The listing builds one solid part. Answer for the finished solid, in the listing's coordinates (mm). Face numbers are marked on the shaded views. A direction names the side the tool comes from. Round coordinates to 2 decimals unless told otherwise and drop trailing zeros. Loops run counter-clockwise (first coordinate to the right, second up) from the corner with the lowest first, then second, coordinate; pieces in that order, holes last. Notation, with made-up numbers: (11.25, 58) -> (49.25, 58) arc R24 ccw to (49.25, 96) -> close; hole circle Ø5 at (-2, 78.5). An arc over 180 degrees is marked (long way). One line per question, with ' | ' between items.
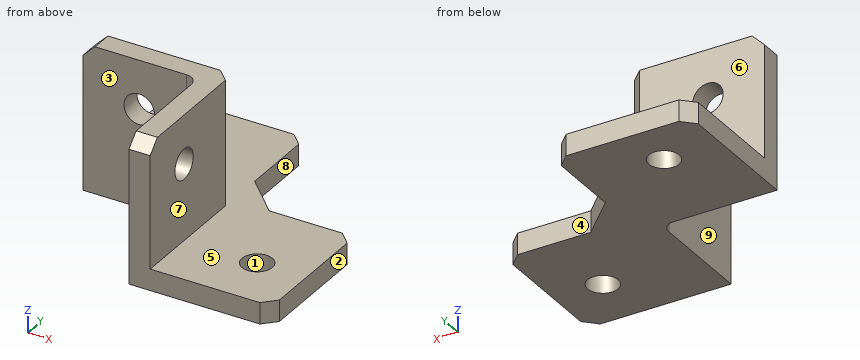
from build123d import *

# Parameters (mm, degrees)
ESQUISSE1_W             = 3.5
ESQUISSE1_H             = 3.5
BOSS_EXTRU_1_DEPTH      = 3.5
ESQUISSE2_W             = 19
ESQUISSE2_H             = 3.5
ESQUISSE2_W_2           = 3.5
ESQUISSE2_H_2           = 19
BOSS_EXTRU_2_DEPTH      = 20.5
ESQUISSE3_R             = 2.5
ENL_V_MAT_EXTRU_2_DEPTH = 3.5
ESQUISSE4_R             = 2.5
ENL_V_MAT_EXTRU_3_DEPTH = 3.5
ESQUISSE5_R             = 2.5
ENL_V_MAT_EXTRU_4_DEPTH = 3.5
ESQUISSE6_R             = 2.5
ENL_V_MAT_EXTRU_5_DEPTH = 3.5
CHANFREIN1_SIZE         = 6
CHANFREIN2_SIZE         = 2
CHANFREIN3_SIZE         = 2
CONG_1_R                = 2


with BuildPart() as part:
    # Esquisse1 → Boss.-Extru.1 (new body)
    with BuildSketch(Plane.XY):
        Polygon((-23.276688067, 13.678057554), (-45.776688067, 13.678057554), (-45.776688067, -9.821942446), (-26.776688067, -9.821942446), (-26.776688067, -6.321942446), (-23.276688067, -6.321942446), align=None)
        with Locations((-25.026688067, -8.071942446)):
            Rectangle(ESQUISSE1_W, ESQUISSE1_H)
        Polygon((-3.276688067, -6.321942446), (-23.276688067, -6.321942446), (-23.276688067, -9.821942446), (-26.776688067, -9.821942446), (-26.776688067, -28.821942446), (-3.276688067, -28.821942446), align=None)
    extrude(amount=BOSS_EXTRU_1_DEPTH)

    # Esquisse2 → Boss.-Extru.2 (add)
    with BuildSketch(Plane.XY.offset(3.5)):
        with Locations((-36.276688067, -8.071942446)):
            Rectangle(ESQUISSE2_W, ESQUISSE2_H)
        with Locations((-25.026688067, -8.071942446)):
            Rectangle(ESQUISSE2_W_2, ESQUISSE2_H)
        with Locations((-25.026688067, -19.321942446)):
            Rectangle(ESQUISSE2_W_2, ESQUISSE2_H_2)
    extrude(amount=BOSS_EXTRU_2_DEPTH)

    # Esquisse3 → Enlèv. mat.-Extru.2 (cut)
    with BuildSketch(Plane(origin=(0, -6.321942446, 0), x_dir=(1, 0, 0), z_dir=(0, 1, 0))):
        with Locations(Location((-36.526688067, -16, 0), (0, 0, 270))):
            Circle(ESQUISSE3_R)
    extrude(amount=-ENL_V_MAT_EXTRU_2_DEPTH, mode=Mode.SUBTRACT)

    # Esquisse4 → Enlèv. mat.-Extru.3 (cut)
    with BuildSketch(Plane(origin=(-23.276688067, 0, 0), x_dir=(0, 0, -1), z_dir=(1, 0, 0))):
        with Locations((-16, -19.571942446)):
            Circle(ESQUISSE4_R)
    extrude(amount=-ENL_V_MAT_EXTRU_3_DEPTH, mode=Mode.SUBTRACT)

    # Esquisse5 → Enlèv. mat.-Extru.4 (cut)
    with BuildSketch(Plane.XY.offset(3.5)):
        with Locations((-36.526688067, 5.678057554)):
            Circle(ESQUISSE5_R)
    extrude(amount=-ENL_V_MAT_EXTRU_4_DEPTH, mode=Mode.SUBTRACT)

    # Esquisse6 → Enlèv. mat.-Extru.5 (cut)
    with BuildSketch(Plane.XY.offset(3.5)):
        with Locations((-11.276688067, -19.571942446)):
            Circle(ESQUISSE6_R)
    extrude(amount=-ENL_V_MAT_EXTRU_5_DEPTH, mode=Mode.SUBTRACT)

    # Chanfrein1
    # the kernel refuses this chamfer: 6 mm, written as the material it adds along each edge
    with BuildSketch(Plane(origin=(-23.276688067, -6.321942446, 0), x_dir=(-0.027495876610586202, 0.9996219169112968, 0), z_dir=(0, 0, 1))) as chanfrein1_piece_1:
        Polygon((CHANFREIN1_SIZE * 0.999621916911, -CHANFREIN1_SIZE * 0.0274958766106), (-CHANFREIN1_SIZE * 0.0274958766106, -CHANFREIN1_SIZE * 0.999621916911), (0, 0), align=None)
    extrude(amount=3.5)

    # Chanfrein2
    chanfrein2_edges = [part.edges().sort_by_distance(p)[0] for p in [
        (-23.276688067, -6.321942446, 13.75),
    ]]
    chamfer(chanfrein2_edges, length=CHANFREIN2_SIZE)

    # Chanfrein3
    chanfrein3_edges = [part.edges().sort_by_distance(p)[0] for p in [
        (-45.776688067, 13.678057554, 1.75),
        (-23.276688067, 13.678057554, 1.75),
        (-3.276688067, -6.321942446, 1.75),
        (-3.276688067, -28.821942446, 1.75),
        (-25.026688067, -28.821942446, 24),
        (-45.776688067, -8.071942446, 24),
    ]]
    chamfer(chanfrein3_edges, length=CHANFREIN3_SIZE)

    # Congé1
    cong_1_edges = [part.edges().sort_by_distance(p)[0] for p in [
        (-26.776688067, -9.821942446, 12),
    ]]
    fillet(cong_1_edges, radius=CONG_1_R)


solid = part.part
Q1. For a pull along Y with two mould halves and no side action, classify the marked faces 1, 2, 3 and 4 as pulls with the +Y half, pulls with the -Y half, needs draft (parallel to the pull), parting line crosses it, or undercut.
Numbers:
face 1: undercut | face 2: needs draft | face 3: pulls with the -Y half | face 4: pulls with the +Y half
Q2. A cutting plane is placed at C-C on z = 2. Give the vertices of the cut face in (x, y).
Numbers:
outline: (-45.78, -9.82) -> (-28.78, -9.82) arc R2 cw to (-26.78, -11.82) -> (-26.78, -28.82) -> (-5.28, -28.82) -> (-3.28, -26.82) -> (-3.28, -8.32) -> (-5.28, -6.32) -> (-17.28, -6.32) -> (-23.28, -0.32) -> (-23.28, 11.68) -> (-25.28, 13.68) -> (-43.78, 13.68) -> (-45.78, 11.68) -> close; hole circle Ø5 at (-36.53, 5.68); hole circle Ø5 at (-11.28, -19.57)
Q3. A cutting plane is placed at B-B on x = -29.5. Give the vertices of the cut face in (y, z).
Numbers:
outline: (-9.82, 0) -> (13.68, 0) -> (13.68, 3.5) -> (-6.32, 3.5) -> (-6.32, 24) -> (-9.82, 24) -> close
Q4. A cutting plane is placed at A-A on z = 16. Give the vertices of the cut face in (x, y), plus the area to 3 significant figures.
Numbers:
outline: (-45.78, -9.82) -> (-39.03, -9.82) -> (-39.03, -6.32) -> (-45.78, -6.32) -> close; (-34.03, -9.82) -> (-28.78, -9.82) arc R2 cw to (-26.78, -11.82) -> (-26.78, -17.07) -> (-23.28, -17.07) -> (-23.28, -8.32) -> (-25.28, -6.32) -> (-34.03, -6.32) -> close; (-26.78, -28.82) -> (-23.28, -28.82) -> (-23.28, -22.07) -> (-26.78, -22.07) -> close | area: 109 mm^2
Q5. For the marked faces 5, 6, 7, 8 and 9, determine the directions among +Z, -Z, +X, -X, +Y, -Y from which every point of the face is accessible in a straight line to the end or side of a thin tool.
Numbers:
face 5: +Z, +X, +Y | face 6: +Z, +X, -X, +Y | face 7: +Z, +X, +Y, -Y | face 8: +Z, -Z, +X, +Y | face 9: +Z, -Z, -X, -Y
Q6. Given pin 1 Ø3 at (y, z) = (5.5, 2) entering from +X; pin 2 Ø6 at (x, z) = (-36.53, 16) entering from -Y; pin 3 Ø13.5 at (y, z) = (-21, 14) entering from -X; pin 4 Ø6 at (x, y) = (-36.53, 5.68) entering from -Z, each flat-ended and moving along its own axis, determine where each tip first touches the part or whether it passes through.
Numbers:
pin 1: x = -23.28 | pin 2: y = -9.82 | pin 3: x = -26.78 | pin 4: z = 0
Q7. Find the intervals of material crossed by line 1 (Z direction, x = -7, y = -14); line 2 (X direction, y = -22, z = 5.5); line 3 (Y direction, x = -32.5, z = 6.25), in increasing order. Write a range as from..to.
Numbers:
line 1: 0..3.5 | line 2: -26.78..-23.28 | line 3: -9.82..-6.32
